The figure shows three views and two pictorial views of one solid part (mm, origin at its lowest corner). Answer the questions. Round coordinates to 2 decimals unless told otherwise and drop trailing zeros. Order: outer loops, then holes, each group sorted by start corner. A loop starts at its lowest first (then second) coordinate and runs counter-clockwise, first axis right, second up. Notation, with made-up numbers: (8, 43) - (49, 43) arc R14 ccw to (49, 60) - close; hole circle Ø1 at (53, 59.25). An arc over 180 degrees is marked (long way). One line per question, with ' | ' between items. Start each with the question number.
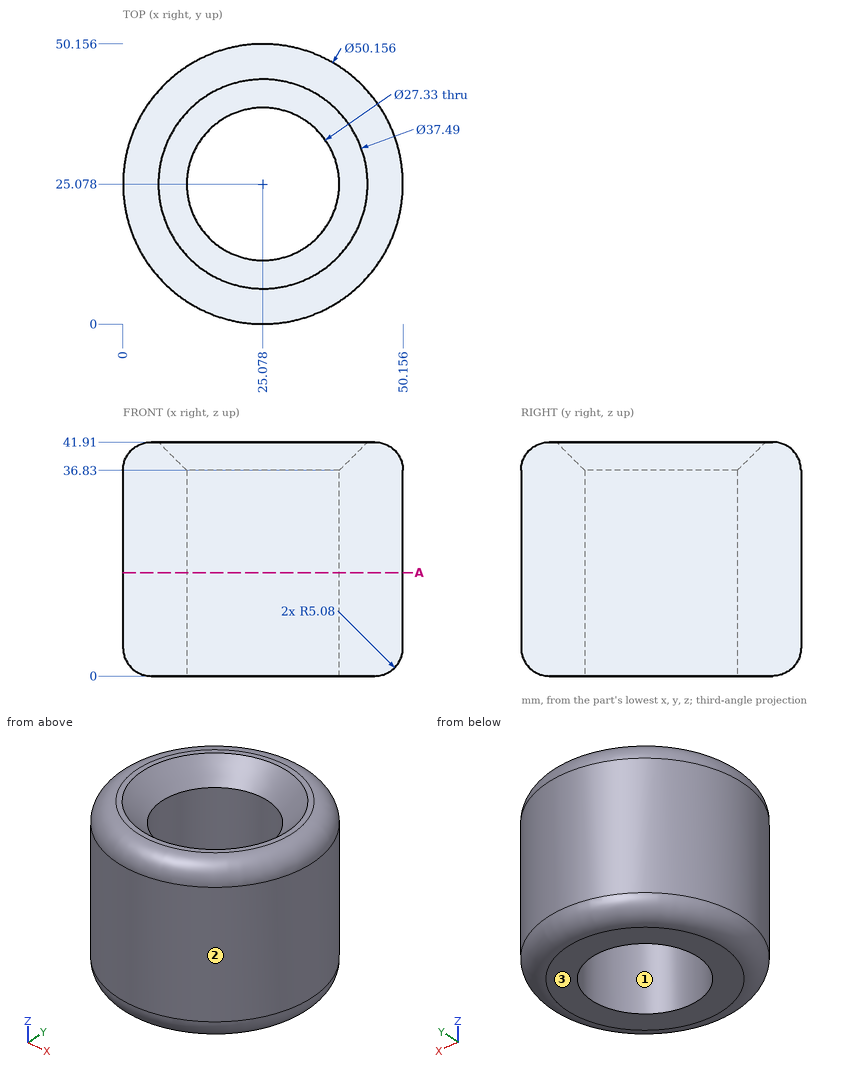
1) Flat-ended cylindrical pins translate along their axes: pin 1 (10 mm diameter, centred on x = 25.5, z = 24, fed in from -Y); pin 2 (8 mm diameter, centred on x = 17.5, z = 13.5, fed in from +Y); pin 3 (8 mm diameter, centred on y = 38.5, z = 33.5, fed in from -X). Find the tip coordinate at first contact, or state that the pin passes through.
2) Section A-A on z = 18.5 is taken. Give the vertices of the cut face in (x, y) (1 decimal), and give its area (3 significant figures).
3) Straight lines are drawn through the part: line 1 (X direction, y = 23, z = 24); line 2 (X direction, y = 29, z = 13); line 3 (Y direction, x = 24, z = 25) (1 decimal). For each, find the intervals that lie inside material, in ascending order.
4) Determine the mould class of the marked faces 1, 2 and 3 for opening direction X: released by +X, released by -X, zero draft, split by the parting line, or undercut.
Recorded:
1) pin 1: stops at y = 0 | pin 2: stops at y = 49.9 | pin 3: stops at x = 1.84
2) outline: circle Ø50.2 at (25.1, 25.1); hole circle Ø27.3 at (25.1, 25.1) | area: 1,390 mm²
3) line 1: x = 0.09 to 11.57, 38.58 to 50.07 | line 2: x = 0.31 to 11.99, 38.17 to 49.85 | line 3: y = 0 to 11.5, 38.7 to 50.1
4) face 1: undercut | face 2: split by the parting line | face 3: zero draft
